Can you work these out from the model? Positions are in its coordinate system, mm. Give positions to 0.01 mm unless a question says otherwise; leave off trailing zeros. Write each loop counter-clockwise with the first axis right and the second up, starting at its lowest first coordinate (ties: lowest second). Pieces come first, ordered by that corner, then holes. Notation, with made-up numbers: (13.25, 76) - (39.25, 76) arc R35 cw to (39.25, 109) - close; hole circle Ø2 at (16, 71.25). An arc over 180 degrees is marked (long way). Use a Markdown table: item, result. Add a question column.
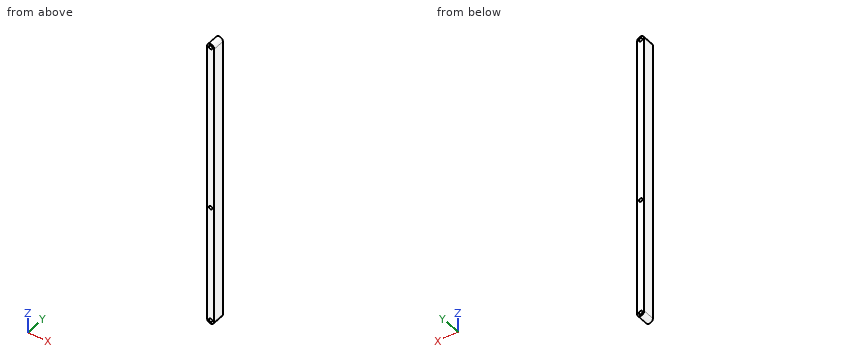
Autodesk Inventor part; units mm, degrees
ref_plane "YZ Plane" through (0, 0, 0) normal (1, 0, 0) x (0, 1, 0)
ref_plane "XZ Plane" through (0, 0, 0) normal (0, 1, 0) x (-1, 0, 0)
ref_plane "XY Plane" through (0, 0, 0) normal (0, 0, 1) x (1, 0, 0)
sketch "Sketch1" plane through (0, 0, 0) normal (0, 1, 0) x (-1, 0, 0)
  line L0 (0, 0) -> (0, -240.109) construction
  line L1 (-3, 0) -> (-3, -240.109)
  line L2 (3, -240.109) -> (3, 0)
  arc A0 (3, 0) -> (-3, 0) centre (0, 0) ccw
  arc A1 (-3, -240.109) -> (3, -240.109) centre (0, -240.109) ccw
  circle A2 centre (0, 0) radius 1.5
  circle A3 centre (0, -240.109) radius 1.5
  circle A4 centre (0, -141.04) radius 1.5
  point P0 (0, -120.0545)
  dimension "d0" = 6
  dimension "d1" = 240.109
  dimension "d2" = 3
  dimension "d3" = 3
  dimension "d6" = 3
  dimension "d7" = 141.04
extrude "Extrusion1" add sketch "Sketch1" along normal blind 10
Q1. I'm going to push a flat-ended pin straight in: P1, Ø2, axis at x = -1.5, y = 5.5, coming from the +Z side. Where does the tip first touch, or does it pass through?
Q2. Suppose I cut it at A-A (y = 4.25). Please give me the cut outline in (x, z).
Q3. Suppose I cut it at B-B (x = 0). Please give me the cut outline in (y, z), and give its area (3 significant figures).
Q4. If I drill on probe 1 along Z at (x, y) = (0, 6.75); probe 2 along Z at (x, y) = (-0.95, 2.5); probe 3 along Z at (x, y) = (2.05, 4.5), over which ranges is the centre line in solid material (lowest first)? Write a range as [from, to].
Derived:
| question | item | result |
|---|---|---|
| 1 | P1 | z = 2.96 |
| 2 | outline | (-3, -240.11) arc R3 ccw to (3, -240.11) - (3, 0) arc R3 ccw to (-3, 0) - close; hole circle Ø3 at (0, -240.11); hole circle Ø3 at (0, -141.04); hole circle Ø3 at (0, 0) |
| 3 | outline | (0, -243.11) - (10, -243.11) - (10, -241.61) - (0, -241.61) - close; (0, -238.61) - (10, -238.61) - (10, -142.54) - (0, -142.54) - close; (0, -139.54) - (10, -139.54) - (10, -1.5) - (0, -1.5) - close; (0, 1.5) - (10, 1.5) - (10, 3) - (0, 3) - close |
| 3 | area | 2,370 mm² |
| 4 | probe 1 | [-243.11, -241.61], [-238.61, -142.54], [-139.54, -1.5], [1.5, 3] |
| 4 | probe 2 | [-242.95, -241.27], [-238.95, -142.2], [-139.88, -1.16], [1.16, 2.85] |
| 4 | probe 3 | [-242.3, 2.19] |
